The drawing under review shows one solid part. Ordinate dimensions are in mm from its lowest x, y, z. Coordinates: 2 decimals unless noted, no trailing zeros. Write each loop counter-clockwise with the first axis right and the second up, starting at its lowest first coordinate (ties: lowest second). Pieces come first, ordered by that corner, then holes. Notation, with made-up numbers: (-13.75, 69) - (34.25, 69) arc R5 cw to (34.25, 76) - close; hole circle Ø1 at (37, 54). An arc over 180 degrees is marked (long way). Put each result on its own line as item: value. Start each with the question number.
Item 1: For pin 1 (0.9 mm diameter, centred on x = 80.5, y = 1.5, fed in from -Z); pin 2 (0.9 mm diameter, centred on y = 2, z = 29, fed in from +X); pin 3 (1.5 mm diameter, centred on x = 5, y = 1, fed in from +Z); pin 4 (10 mm diameter, centred on x = 119, z = 25, fed in from -Y), all flat-tipped, find the tip position at first contact; note any pin that passes through.
Item 2: To check wall thickness, follow L1, parallel to Z at x = 46, y = 2.25. State the ranges of the line that lie inside material, in increasing order. Write a range as [from, to].
Item 3: Consider section A-A on x = 80. Give the boundary of the cut face in (y, z).
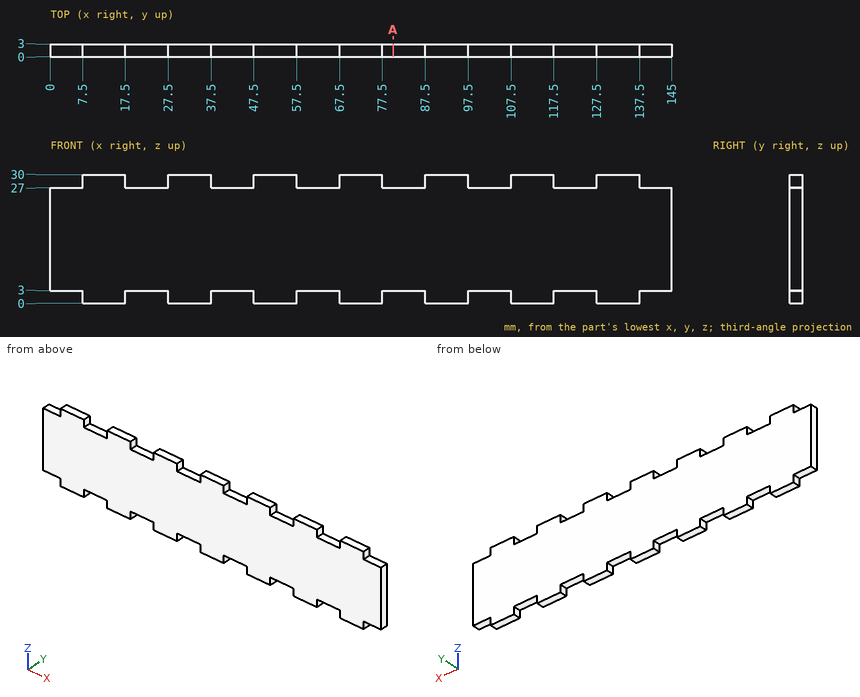
Report:
1. pin 1: z = 3
1. pin 2: x = 137.5
1. pin 3: z = 27
1. pin 4: y = 0
2. L1: [3, 27]
3. outline: (0, 3) - (3, 3) - (3, 27) - (0, 27) - close
